Source: CAD feature listing. Evaluate the final solid. Frame: model axes, mm. Face numbers are marked on the shaded views. A direction names the side the tool comes from. Round coordinates to 2 decimals unless told otherwise and drop trailing zeros. Order: outer loops, then holes, each group sorted by start corner. A loop starts at its lowest first (then second) coordinate and runs counter-clockwise, first axis right, second up. Notation, with made-up numbers: (28, 48.25) -> (70, 48.25) arc R21 cw to (70, 52.25) -> close; hole circle Ø10 at (23, 84). An arc over 180 degrees is marked (long way). Write item = value, one per line. Start each with the question number.
(1) Ray query, line 1 (X direction, y = 74.5, z = 21) (3 decimals); line 2 (Y direction, x = -59.5, z = -7.5). Return the intervals inside material, ascending.
(2) Cut plane B-B on x = 0. Return the cut outline in (y, z), then the cut area to 3 significant figures.
(3) Cut plane D-D on y = 45.5. Return the cut outline in (x, z) (3 decimals), then the cut area to 3 significant figures.
(4) Cut plane A-A on y = 12.7. Return the cut outline in (x, z) (3 decimals), then the cut area to 3 significant figures.
(5) Cut plane C-C on z = 0. Return the cut outline in (x, y) (3 decimals), then the cut area to 3 significant figures.
(6) Reachability of the marked faces 1 and 2 from +Z, -Z, +X, -X, +Y, -Y: full face, straight path, thin tool, end or side. Return the list, or none.
(7) Contact query for flat-ended pins moving along their axis: pin 1 Ø3 at (y, z) = (52.5, -0.5) entering from +X (3 decimals); pin 2 Ø10 at (x, z) = (-39.5, 41) entering from +Y; pin 3 Ø6 at (y, z) = (138.5, -1) entering from -X (3 decimals). Output: stop coordinate, or through.
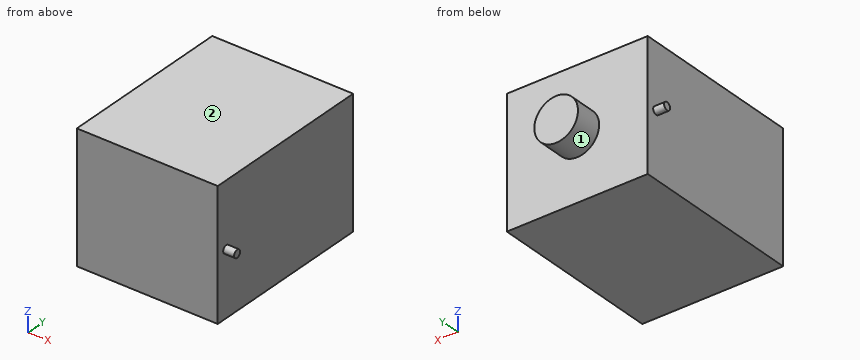
from build123d import *

# Parameters (mm, degrees)
SKETCH1_W           = 163.83
SKETCH1_H           = 149.352
BOSS_EXTRUDE1_DEPTH = 203.2
SKETCH2_R           = 25.4
BOSS_EXTRUDE2_DEPTH = 31.75
SKETCH3_R           = 4.5
BOSS_EXTRUDE3_DEPTH = 12.7
SKETCH5_R           = 4.5
BOSS_EXTRUDE4_DEPTH = 12.7


with BuildPart() as part:
    # Sketch1 → Boss-Extrude1 (new body)
    with BuildSketch(Plane(origin=(0, 0, 0), x_dir=(1, 0, 0), z_dir=(0, 1, 0))):
        Rectangle(SKETCH1_W, SKETCH1_H)
    extrude(amount=BOSS_EXTRUDE1_DEPTH)

    # Sketch2 → Boss-Extrude2 (add)
    with BuildSketch(Plane(origin=(0, 203.2, 0), x_dir=(1, 0, 0), z_dir=(0, 1, 0))):
        with Locations(Location((0, 0, 0), (0, 0, 270))):
            Circle(SKETCH2_R)
    extrude(amount=BOSS_EXTRUDE2_DEPTH)

    # Sketch3 → Boss-Extrude3 (add)
    with BuildSketch(Plane.ZY.offset(81.915)):
        with Locations(Location((0, 190.5, 0), (0, 0, 180))):
            Circle(SKETCH3_R)
    extrude(amount=BOSS_EXTRUDE3_DEPTH)

    # Sketch5 → Boss-Extrude4 (add)
    with BuildSketch(Plane(origin=(81.915, 0, 0), x_dir=(0, 0, -1), z_dir=(1, 0, 0))):
        with Locations(Location((0, 12.7, 0), (0, 0, 180))):
            Circle(SKETCH5_R)
    extrude(amount=BOSS_EXTRUDE4_DEPTH)


solid = part.part
Evaluation:
q1.line_1 = -81.915 to 81.915
q1.line_2 = 0 to 203.2
q2.outline = (0, -74.68) -> (203.2, -74.68) -> (203.2, -25.4) -> (234.95, -25.4) -> (234.95, 25.4) -> (203.2, 25.4) -> (203.2, 74.68) -> (0, 74.68) -> close
q2.area = 32,000 mm^2
q3.outline = (-81.915, -74.676) -> (81.915, -74.676) -> (81.915, 74.676) -> (-81.915, 74.676) -> close
q3.area = 24,500 mm^2
q4.outline = (-81.915, -74.676) -> (81.915, -74.676) -> (81.915, -4.5) -> (94.615, -4.5) -> (94.615, 4.5) -> (81.915, 4.5) -> (81.915, 74.676) -> (-81.915, 74.676) -> close
q4.area = 24,600 mm^2
q5.outline = (-94.615, 186) -> (-81.915, 186) -> (-81.915, 0) -> (81.915, 0) -> (81.915, 8.2) -> (94.615, 8.2) -> (94.615, 17.2) -> (81.915, 17.2) -> (81.915, 203.2) -> (25.4, 203.2) -> (25.4, 234.95) -> (-25.4, 234.95) -> (-25.4, 203.2) -> (-81.915, 203.2) -> (-81.915, 195) -> (-94.615, 195) -> close
q5.area = 35,100 mm^2
q6.face_1 = +Y
q6.face_2 = +Z, +X, -X, +Y, -Y
q7.pin_1 = 81.915
q7.pin_2 = 203.2
q7.pin_3 = -81.915
